Geometry check sheet. Reference: the model listing, model coordinates, mm. Face numbers are marked on the shaded views. Give positions to 0.01 mm unless a question says otherwise; leave off trailing zeros. Loops run counter-clockwise (first coordinate to the right, second up) from the corner with the lowest first, then second, coordinate; pieces in that order, holes last. Notation, with made-up numbers: (71.5, 39) -> (103.5, 39) arc R25 ccw to (103.5, 76) -> close; hole circle Ø2 at (65, -5.75). An arc over 180 degrees is marked (long way). Write item = value, one per line. Start each with the question number.
```python
from build123d import *

# Parameters (mm, degrees)
F0_W     = 304.8
F0_H     = 127
F1_DEPTH = 19.05
F2_R     = 30.1625
F2_R_2   = 23.914231
F3_DEPTH = 152.4


with BuildPart() as f1:
    # F0 (on Top) → F1 (new body)
    with BuildSketch(Plane.XY):
        Rectangle(F0_W, F0_H)
    extrude(amount=F1_DEPTH)

    # F2 (on face) → F3 (join)
    with BuildSketch(Plane.XY.offset(19.05)):
        with Locations((-114.3, 0)):
            Circle(F2_R)
        with Locations((-114.3, 0)):
            Circle(F2_R_2, mode=Mode.SUBTRACT)
    extrude(amount=F3_DEPTH)


solid = f1.part
```
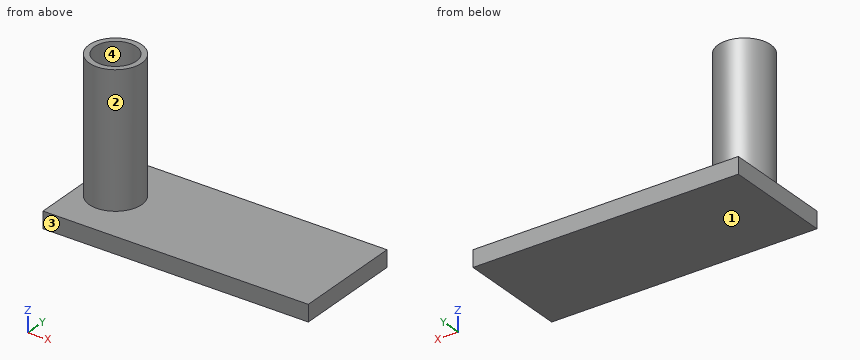
1) Draft check along Y on the marked faces 1, 2, 3 and 4. Enter one of: released by +Y, released by -Y, zero draft, split by the parting line, or undercut.
2) Section check B-B (y = 0). Enter the section's corners in (x, z).
3) Thickness scan on line 1 (Y direction, x = -114.3, z = 102); line 2 (Z direction, x = 22.5, y = 55); line 3 (X direction, y = -19, z = 45.5). Record the ranges inside material, lowest first.
4) Section check D-D (x = -61). Enter the section's corners in (y, z).
5) Section check A-A (x = -114.3). Enter the section's corners in (y, z).
6) Depth check by flat-ended pin: pin 1 Ø1 at (x, y) = (118.5, -17.5) entering from +Z; pin 2 Ø1.5 at (y, z) = (-20.5, 61) entering from +X; pin 3 Ø6 at (x, y) = (-44, -44) entering from -Z; pin 4 Ø8 at (y, z) = (20, 59.5) entering from -X. Enter the tip coordinate at first touch or a pass-through.
7) Section check C-C (z = 125.5). Enter the section's corners in (x, y) (1 decimal), plus the area to 3 significant figures.
Check result:
q1.face_1 = zero draft
q1.face_2 = split by the parting line
q1.face_3 = released by -Y
q1.face_4 = undercut
q2.outline = (-152.4, 0) -> (152.4, 0) -> (152.4, 19.05) -> (-84.14, 19.05) -> (-84.14, 171.45) -> (-90.39, 171.45) -> (-90.39, 19.05) -> (-138.21, 19.05) -> (-138.21, 171.45) -> (-144.46, 171.45) -> (-144.46, 19.05) -> (-152.4, 19.05) -> close
q3.line_1 = -30.16 to -23.91, 23.91 to 30.16
q3.line_2 = 0 to 19.05
q3.line_3 = -137.73 to -128.82, -99.78 to -90.87
q4.outline = (-63.5, 0) -> (63.5, 0) -> (63.5, 19.05) -> (-63.5, 19.05) -> close
q5.outline = (-63.5, 0) -> (63.5, 0) -> (63.5, 19.05) -> (30.16, 19.05) -> (30.16, 171.45) -> (23.91, 171.45) -> (23.91, 19.05) -> (-23.91, 19.05) -> (-23.91, 171.45) -> (-30.16, 171.45) -> (-30.16, 19.05) -> (-63.5, 19.05) -> close
q6.pin_1 = 19.05
q6.pin_2 = -91.5
q6.pin_3 = 0
q6.pin_4 = -139.87
q7.outline = circle Ø60.3 at (-114.3, 0); hole circle Ø47.8 at (-114.3, 0)
q7.area = 1,060 mm2
